Part print with two shaded views. Sizes in mm from the minimum x, y, z corner. Round coordinates to 2 decimals unless told otherwise and drop trailing zeros. Write each loop counter-clockwise with the first axis right and the second up, starting at its lowest first coordinate (ties: lowest second). Pieces come first, ordered by that corner, then holes. Notation, with made-up numbers: (9.25, 53.5) -> (15.25, 53.5) arc R24 cw to (15.25, 77.5) -> close; hole circle Ø11 at (-31.5, 30.5). An arc over 180 degrees is marked (long way). Answer in a Markdown table with one row per item.
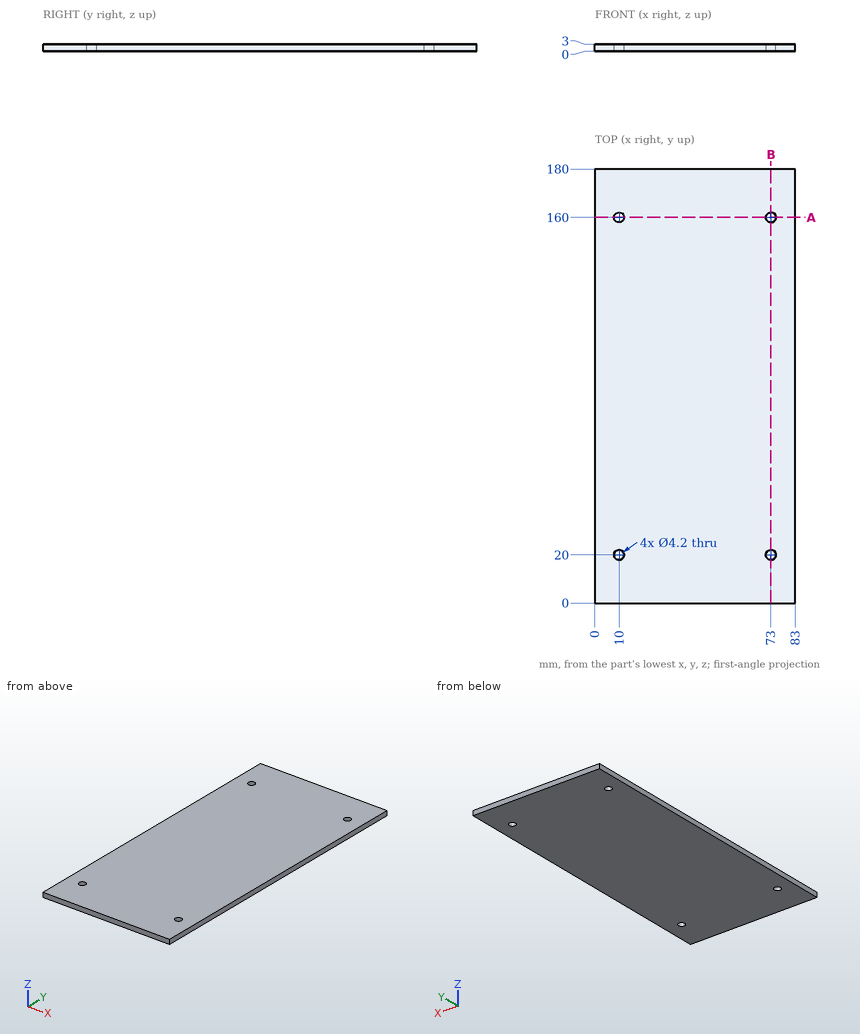
Q1. Saw through at A-A on y = 160. Write the cut outline in (x, z), plus the area to 3 significant figures.
A:
| item | result |
|---|---|
| outline | (0, 0) -> (7.9, 0) -> (7.9, 3) -> (0, 3) -> close; (12.1, 0) -> (70.9, 0) -> (70.9, 3) -> (12.1, 3) -> close; (75.1, 0) -> (83, 0) -> (83, 3) -> (75.1, 3) -> close |
| area | 224 mm² |
Q2. Saw through at B-B on x = 73. Write the cut outline in (y, z).
A:
| item | result |
|---|---|
| outline | (0, 0) -> (17.9, 0) -> (17.9, 3) -> (0, 3) -> close; (22.1, 0) -> (157.9, 0) -> (157.9, 3) -> (22.1, 3) -> close; (162.1, 0) -> (180, 0) -> (180, 3) -> (162.1, 3) -> close |
Q3. Wall check: line 1 (X direction, y = 20, z = 2.2); line 2 (Y direction, x = 73, z = 0.75); line 3 (X direction, y = 18.5, z = 0.7). Give the ranges that are in metal, low to high. Write a range as [from, to].
A:
| item | result |
|---|---|
| line 1 | [0, 7.9], [12.1, 70.9], [75.1, 83] |
| line 2 | [0, 17.9], [22.1, 157.9], [162.1, 180] |
| line 3 | [0, 8.53], [11.47, 71.53], [74.47, 83] |
